Autodesk Inventor part; units mm, degrees
ref_plane "YZ Plane" through (0, 0, 0) normal (1, 0, 0) x (0, 1, 0)
ref_plane "XZ Plane" through (0, 0, 0) normal (0, 1, 0) x (-1, 0, 0)
ref_plane "XY Plane" through (0, 0, 0) normal (0, 0, 1) x (1, 0, 0)
sketch "Sketch1" plane through (0, 0, 0) normal (1, 0, 0) x (0, 1, 0)
  line L0 (0, -2) -> (5, -2)
  line L1 (5, -2) -> (5, -19)
  line L2 (5, -19) -> (35, -19)
  line L3 (35, -19) -> (35, -23)
  line L4 (35, -23) -> (5, -23)
  line L5 (5, -23) -> (5, -40)
  line L6 (5, -40) -> (0, -40)
  line L7 (0, -40) -> (0, -2)
  line L8 (-7, 0) -> (42, 0)
  point P0 (0, 0)
  dimension "d0" = 35
  dimension "d1" = 2
  dimension "d2" = 5
  dimension "d3" = 19
  dimension "d4" = 23
  dimension "d5" = 40
revolve "Revolution1" add sketch "Sketch1" angle 360 about axis through (0, -10, 0) along (0, 1, 0)
properties material "ABS Plastic"
Source: CAD feature listing. Evaluate the final solid. Frame: model axes, mm. A direction names the side the tool comes from. Give positions to 0.01 mm unless a question says otherwise; leave off trailing zeros. Loops run counter-clockwise (first coordinate to the right, second up) from the corner with the lowest first, then second, coordinate; pieces in that order, holes last. Notation, with made-up numbers: (56, 66.25) -> (83, 66.25) arc R29 cw to (83, 87.25) -> close; hole circle Ø8 at (48, -36.75). An arc over 180 degrees is marked (long way). Use a Markdown table: item, result. Add a question column.
(1) First-contact query: pin 1 Ø10 at (y, z) = (20, 5) entering from +X; pin 2 Ø2 at (x, z) = (-18.5, 31) entering from +Y; pin 3 Ø4 at (x, y) = (-5.5, 29) entering from -Z. Flat tips, straight axial feed; report the tip coordinate or a pass-through.
(2) Access query for faces 4 (the face through (22.804, 19.79, 2.994)), 5 (the face through (2, 3, 0)). Directions: +Z, -Z, +X, -X, +Y, -Y. A direction counts if a zero-diameter tool reaches every point of the face in a straight line with its end or side. Return the directions, or none.
(3) Section query D-D (x = -13). Output: boundary loops of the cut face in (y, z), then the cut area to 3 significant figures.
(4) Section query B-B (z = 0). Output: boundary loops of the cut face in (x, y).
(5) Pull-direction query (X, two-part tool) for faces 1 (the face through (-39.05, 2.46, 8.67)), 2 (the face through (-1, 0, -8)), 3 (the face through (4, 5, 0)); classes: +X half, -X half, draft (parallel to the pull), parting line (faces both ways), or undercut.
(6) Section query A-A (x = 0). Output: boundary loops of the cut face in (y, z).
(7) Ray query, line 1 (X direction, y = 16.5, z = 0); line 2 (X direction, y = 3.25, z = 0); line 3 (Z direction, x = 0.5, y = 33). Return the intervals inside material, ascending.
(8) Section query C-C (y = 28). Output: boundary loops of the cut face in (x, z).
Checked values:
| question | item | result |
|---|---|---|
| 1 | pin 1 | x = 23 |
| 1 | pin 2 | y = 5 |
| 1 | pin 3 | z = -22.73 |
| 2 | face 4 | +Y |
| 2 | face 5 | +Y, -Y |
| 3 | outline | (0, -37.83) -> (5, -37.83) -> (5, -18.97) -> (35, -18.97) -> (35, -13.86) -> (5, -13.86) -> (5, 13.86) -> (35, 13.86) -> (35, 18.97) -> (5, 18.97) -> (5, 37.83) -> (0, 37.83) -> close |
| 3 | area | 685 mm^2 |
| 4 | outline | (-40, 0) -> (-2, 0) -> (-2, 5) -> (-19, 5) -> (-19, 35) -> (-23, 35) -> (-23, 5) -> (-40, 5) -> close; (2, 0) -> (40, 0) -> (40, 5) -> (23, 5) -> (23, 35) -> (19, 35) -> (19, 5) -> (2, 5) -> close |
| 5 | face 1 | parting line |
| 5 | face 2 | draft |
| 5 | face 3 | undercut |
| 6 | outline | (0, -40) -> (5, -40) -> (5, -23) -> (35, -23) -> (35, -19) -> (5, -19) -> (5, -2) -> (0, -2) -> close; (0, 2) -> (5, 2) -> (5, 19) -> (35, 19) -> (35, 23) -> (5, 23) -> (5, 40) -> (0, 40) -> close |
| 7 | line 1 | -23 to -19, 19 to 23 |
| 7 | line 2 | -40 to -2, 2 to 40 |
| 7 | line 3 | -22.99 to -18.99, 18.99 to 22.99 |
| 8 | outline | circle Ø46 at (0, 0); hole circle Ø38 at (0, 0) |
